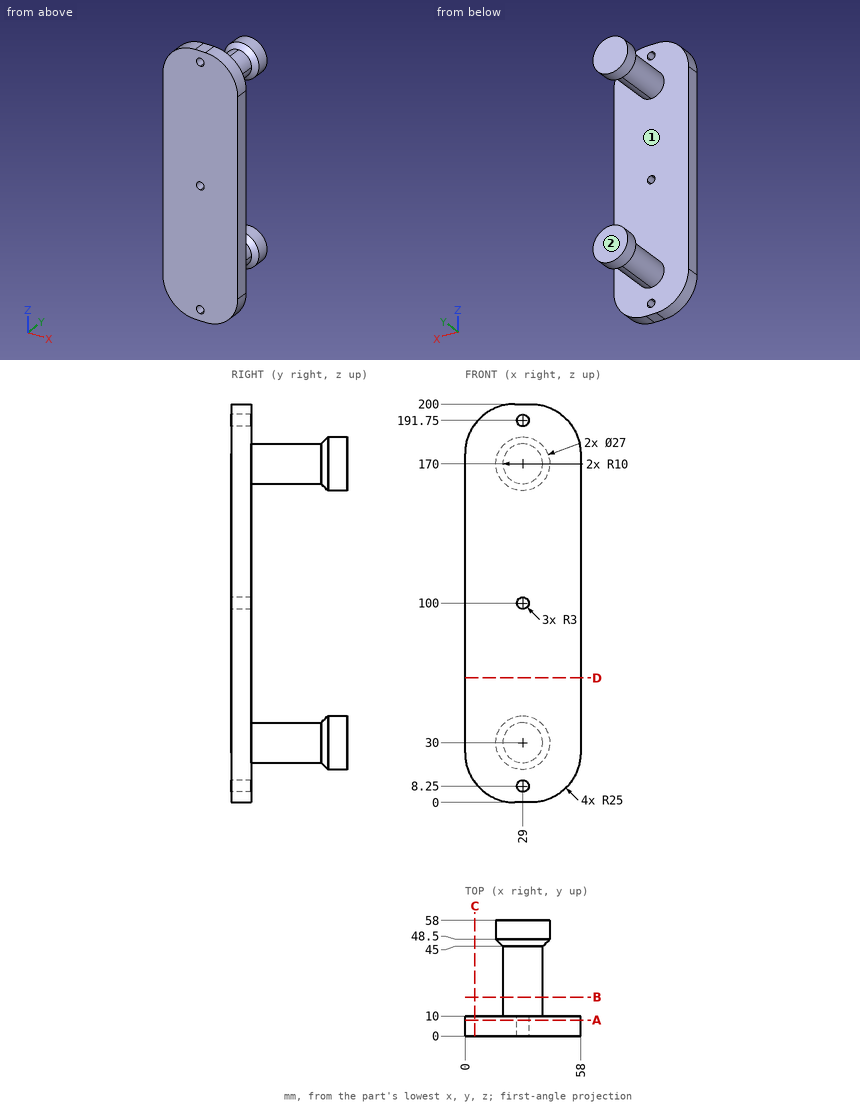
Part print with two shaded views. Sizes in mm from the minimum x, y, z corner. Give positions to 0.01 mm unless a question says otherwise; leave off trailing zeros. Order: outer loops, then holes, each group sorted by start corner. A loop starts at its lowest first (then second) coordinate and runs counter-clockwise, first axis right, second up.
1) Saw through at B-B, the plane y = 19.5. Write the cut outline in (x, z).
2) Wall check: probe 1 along Z at (x, y) = (28.5, 32); probe 2 along Y at (x, z) = (8.5, 60); probe 3 along Z at (x, y) = (23.5, 43). Give the ranges that are in metal, low to high.
3) Mould opens along Z. For the marked faces 1 and 2 say: +Z half, -Z half, draft (parallel to the pull), parting line (faces both ways), or undercut.
4) Saw through at A-A, the plane y = 8. Write the cut outline in (x, z).
5) Saw through at C-C, the plane x = 5. Write the cut outline in (y, z).
6) Saw through at D-D, the plane z = 62.5. Write the cut outline in (x, y).
7) Pin check, flat tips, straight feed: pin 1 (5 mm diameter, centred on y = 33.5, z = 22, fed in from -X); pin 2 (6 mm diameter, centred on y = 21.5, z = 178, fed in from -X); pin 3 (10 mm diameter, centred on x = 41.5, y = 12, fed in from -Z). Stop position of each tip, or through.
Computed:
1. outline: circle Ø20 at (29, 30); circle Ø20 at (29, 170)
2. probe 1: z = 20.01 to 39.99, 160.01 to 179.99
2. probe 2: y = 0 to 10
2. probe 3: z = 21.65 to 38.35, 161.65 to 178.35
3. face 1: undercut
3. face 2: draft
4. outline: (0, 25) arc R25 ccw to (25, 0) - (33, 0) arc R25 ccw to (58, 25) - (58, 175) arc R25 ccw to (33, 200) - (25, 200) arc R25 ccw to (0, 175) - close; hole circle Ø6 at (29, 8.25); hole circle Ø6 at (29, 100); hole circle Ø6 at (29, 191.75)
5. outline: (0, 10) - (10, 10) - (10, 190) - (0, 190) - close
6. outline: (0, 0) - (58, 0) - (58, 10) - (0, 10) - close
7. pin 1: stops at x = 20.65
7. pin 2: stops at x = 20.34
7. pin 3: stops at z = 0.31
